Read the model definition and answer for the solid it produces. Units are mm, in the model's axes. A direction names the side the tool comes from. Coordinates: 2 decimals unless noted, no trailing zeros. Loops run counter-clockwise (first coordinate to the right, second up) from the corner with the lowest first, then second, coordinate; pieces in that order, holes last. Notation, with made-up numbers: (46, -17) -> (99, -17) arc R26 cw to (99, -1) -> close; hole circle Ø6 at (-23, 73). An arc over 180 degrees is marked (long way). Answer as a JSON object with one key per item and string values. Group by question number.
Q1. Each of these flat-tipped pins is pushed along its axis until it touches: P1, Ø5, axis at x = -10, z = 6.5, coming from the +Y side; P2, Ø8, axis at y = 6, z = 8.5, coming from the -X side. Where does it stop, or does it pass through?
Q2. The part is cut by section D-D on y = 9.5. Write down the section's boundary in (x, z).
Q3. The part is cut by section B-B on x = -18.5. Write down the section's boundary in (y, z), and give its area (3 significant figures).
Q4. For faces 1 (the cylindrical face through (-4, -1, 15)), 2 (the flat face through (0, 4, 15)), 3 (the cylindrical face through (0.9, 5.42, 29.14)), 4 (the cylindrical face through (0.9, 5.42, 0.86)), 5 (the flat face through (15, 0, 15)), determine the directions among +Z, -Z, +X, -X, +Y, -Y from which every point of the face is accessible in a straight line to the end or side of a thin tool.
Q5. Determine the mould class of faces 6 (the flat face through (2, -3, 15)), 7 (the flat face through (3, -1, 30)), 8 (the cylindrical face through (-27, -1, 15)) for opening direction Z: released by +Z, released by -Z, zero draft, split by the parting line, or undercut.
Q6. Straight lines are drawn through the part: line 1 along Y through (x, z) = (-10.5, 2); line 2 along Z through (x, y) = (-14, -0.75); line 3 along X through (y, z) = (-0.5, 9.5). For each, find the intervals that lie inside material, in ascending order. Write a range as [from, to].
Q7. The part is cut by section C-C on y = 2. Write down the section's boundary in (x, z).
Q8. The part is cut by section A-A on z = 15. Write down the section's boundary in (x, y).
from build123d import *

# Parameters (mm, degrees)
PAD_DEPTH    = 30
POCKET_DEPTH = 5
FILLET_R     = 3
FILLET001_R  = 10


with BuildPart() as part:
    # Sketch → Pad (new body)
    with BuildSketch(Plane.XY):
        Polygon((-34, -3), (26, -3), (26, 11), (19, 11), (22.565685, 0), (7.565685, 0), (5, 11), (0, 11), (0, 0), (-34, 0), align=None)
    extrude(amount=PAD_DEPTH)

    # Sketch001 → Pocket (cut)
    with BuildSketch(Plane(origin=(0, 0, 0), x_dir=(-1, 0, 0), z_dir=(0, 1, 0))):
        with BuildLine():
            ThreePointArc((15, 26), (4, 15), (15, 4))
            Line((15, 4), (16, 4))
            ThreePointArc((16, 4), (27, 15), (16, 26))
            Line((15, 26), (16, 26))
        make_face()
    extrude(amount=-POCKET_DEPTH, mode=Mode.SUBTRACT)

    # Fillet
    fillet_edges = [part.edges().sort_by_distance(p)[0] for p in [
        (0, 11, 15),
        (0, 5.5, 30),
        (0, 5.5, 0),
        (26, 4, 0),
        (26, 11, 15),
        (26, 4, 30),
    ]]
    fillet(fillet_edges, radius=FILLET_R)

    # Fillet001
    fillet001_edges = [part.edges().sort_by_distance(p)[0] for p in [
        (-34, -1.5, 0),
        (-34, -1.5, 30),
    ]]
    fillet(fillet001_edges, radius=FILLET001_R)


solid = part.part
Final values:
{
 "1": {"P1": "stops at y = 0", "P2": "stops at x = 0"},
 "2": {"outline": "(0.4, 1.5) arc R3 ccw to (3, 0) -> (5.35, 0) -> (5.35, 30) -> (3, 30) arc R3 ccw to (0.4, 28.5) -> close; (19.49, 0) -> (23, 0) arc R3 ccw to (25.6, 1.5) -> (25.6, 28.5) arc R3 ccw to (23, 30) -> (19.49, 30) -> close"},
 "3": {"outline": "(-3, 0) -> (0, 0) -> (0, 4.29) -> (-3, 4.29) -> close; (-3, 25.71) -> (0, 25.71) -> (0, 30) -> (-3, 30) -> close", "area": "25.7 mm2"},
 "4": {"face 1": "+Y, -Y", "face 2": "+Z, -Z, -X, +Y", "face 3": "+Z, -X, +Y", "face 4": "-Z, -X, +Y", "face 5": "+Z, -Z"},
 "5": {"face 6": "zero draft", "face 7": "released by +Z", "face 8": "undercut"},
 "6": {"line 1": "y = [-3, 0]", "line 2": "z = [0, 4.05], [25.95, 30]", "line 3": "x = [-33.99, -25.53], [-5.47, 26]"},
 "7": {"outline": "(0, 3) arc R3 ccw to (3, 0) -> (7.1, 0) -> (7.1, 30) -> (3, 30) arc R3 ccw to (0, 27) -> close; (21.92, 0) -> (23, 0) arc R3 ccw to (26, 3) -> (26, 27) arc R3 ccw to (23, 30) -> (21.92, 30) -> close"},
 "8": {"outline": "(-34, -3) -> (-27, -3) -> (-27, 0) -> (-34, 0) -> close; (-4, -3) -> (26, -3) -> (26, 8) arc R3 ccw to (23, 11) -> (19, 11) -> (22.57, 0) -> (7.57, 0) -> (5, 11) -> (3, 11) arc R3 ccw to (0, 8) -> (0, 0) -> (-4, 0) -> close"}
}
